Could you check a few things on this model? Use its own coordinates, in mm. A direction names the side the tool comes from. Round coordinates to 2 decimals unless told otherwise and drop trailing zeros. Loops run counter-clockwise (first coordinate to the right, second up) from the corner with the lowest first, then second, coordinate; pieces in that order, holes last. Notation, with made-up numbers: (44.5, -33.5) -> (70.5, -33.5) arc R14 cw to (70.5, -25.5) -> close; hole circle Ø10 at (-29, 57.25). An arc over 180 degrees is marked (long way). Put each result on its own line as item: value. Start each with the question number.
1. Imagine slicing it at B-B, the plane y = 20. Please give me the cut outline in (x, z), and give its area (3 significant figures).
2. I need wall thicknesses on line 1 (Y direction, x = 0, z = 0.5); line 2 (X direction, y = -3.5, z = 0.9); line 3 (X direction, y = 13.5, z = 0.7). Which ranges of each line are inside material? Lowest first, please. Write a range as [from, to].
3. I'm going to push a flat-ended pin straight in: P1, Ø4, axis at x = -11.76, y = -16.18, coming from the -Z side. Where does the tip first touch, or does it pass through?
4. Imagine slicing it at D-D, the plane z = 0.6. Count the separate pieces of the cut face and the enclosed holes in it, and give its area (3 significant figures).
5. If we mould it in two halves opening along X, with no side actions, what happens to faces 5 (the cylindrical face through (-17.156, -12.788, 0.493)), 6 (the cylindrical face through (17.369, 12.376, 0.493)), 7 (the cylindrical face through (6.363, 20.43, 0.493))? For each: pulls with the +X half, pulls with the -X half, needs draft (parallel to the pull), parting line crosses it, or undercut.
6. Which directions (+Z, -Z, +X, -X, +Y, -Y) give clear straight access to the entire face, cutting with the end or side of a thin tool? Please do faces 1 (the cylindrical face through (-17.464, 12.365, 0.493)), 2 (the flat face through (-6.925, 27.045, 0.493)), 3 (the flat face through (10.33, -26.04, 0.49)), 4 (the flat face through (6.95, 27.14, 0.49)).
7. Imagine slicing it at A-A, the plane x = 0. Please give me the cut outline in (y, z), and give its area (3 significant figures).
8. Imagine slicing it at C-C, the plane x = 22.5. Please give me the cut outline in (y, z), and give its area (3 significant figures).
```python
from build123d import *

# Parameters (mm, degrees)
SKETCH_1_R      = 12.9
SKETCH_1_R_2    = 1.5
EXTRUDE_1_DEPTH = 1


with BuildPart() as part:
    # 草图1 → 凸台-拉伸1 (new body)
    with BuildSketch(Plane.XY):
        with BuildLine():
            Line((-24.208730048, -20.05461018), (-18.863150132, -15.626310092))
            ThreePointArc((-18.863150132, -15.626310092), (-17.146898547, -12.74106365), (-17.642285858, -9.420708556))
            ThreePointArc((-17.642285858, -9.420708556), (-19.021130326, -6.180339887), (-19.810262634, -2.748362124))
            ThreePointArc((-19.810262634, -2.748362124), (-21.361141637, 0.229042931), (-24.445523644, 1.554468964))
            Line((-24.445523644, 1.554468964), (-31.373078125, 1.994985952))
            ThreePointArc((-31.373078125, 1.994985952), (-32.788486399, 2.717684101), (-33.230039203, 4.244348542))
            ThreePointArc((-33.230039203, 4.244348542), (-31.860393296, 10.352069312), (-29.378431918, 16.098376876))
            ThreePointArc((-29.378431918, 16.098376876), (-28.123857351, 17.073936127), (-26.55397669, 16.826655102))
            Line((-26.55397669, 16.826655102), (-20.690537997, 13.111126473))
            ThreePointArc((-20.690537997, 13.111126473), (-17.41615466, 12.370464403), (-14.41139241, 13.867651885))
            ThreePointArc((-14.41139241, 13.867651885), (-11.755705046, 16.180339888), (-8.735555524, 17.991388765))
            ThreePointArc((-8.735555524, 17.991388765), (-6.383123013, 20.386431107), (-6.075694405, 23.729431883))
            Line((-6.075694405, 23.729431883), (-7.797469917, 30.45405495))
            ThreePointArc((-7.797469917, 30.45405495), (-7.547528343, 32.023514221), (-6.232031499, 32.915221151))
            ThreePointArc((-6.232031499, 32.915221151), (0, 33.5), (6.232031499, 32.915221151))
            ThreePointArc((6.232031499, 32.915221151), (7.547528343, 32.023514221), (7.797469917, 30.45405495))
            Line((7.797469917, 30.45405495), (6.075694405, 23.729431883))
            ThreePointArc((6.075694405, 23.729431883), (6.383123013, 20.386431107), (8.735555524, 17.991388765))
            ThreePointArc((8.735555524, 17.991388765), (11.755705046, 16.180339887), (14.41139241, 13.867651885))
            ThreePointArc((14.41139241, 13.867651885), (17.41615466, 12.370464403), (20.690537997, 13.111126473))
            Line((20.690537997, 13.111126473), (26.55397669, 16.826655102))
            ThreePointArc((26.55397669, 16.826655102), (28.123857351, 17.073936127), (29.378431918, 16.098376876))
            ThreePointArc((29.378431918, 16.098376876), (31.860393296, 10.352069312), (33.230039203, 4.244348542))
            ThreePointArc((33.230039203, 4.244348542), (32.788486399, 2.717684101), (31.373078125, 1.994985952))
            Line((31.373078125, 1.994985952), (24.445523644, 1.554468964))
            ThreePointArc((24.445523644, 1.554468964), (21.361141637, 0.229042931), (19.810262634, -2.748362124))
            ThreePointArc((19.810262634, -2.748362124), (19.021130326, -6.180339888), (17.642285858, -9.420708556))
            ThreePointArc((17.642285858, -9.420708556), (17.146898547, -12.74106365), (18.863150132, -15.626310092))
            Line((18.863150132, -15.626310092), (24.208730048, -20.05461018))
            ThreePointArc((24.208730048, -20.05461018), (24.929028081, -21.471241373), (24.388900961, -22.965877077))
            ThreePointArc((24.388900961, -22.965877077), (19.690805952, -27.102069312), (14.305262176, -30.292069492))
            ThreePointArc((14.305262176, -30.292069492), (12.71687069, -30.343893076), (11.592158696, -29.221085825))
            Line((11.592158696, -29.221085825), (9.03247008, -22.768717229))
            ThreePointArc((9.03247008, -22.768717229), (6.818788557, -20.244874791), (3.50786011, -19.689969971))
            ThreePointArc((3.50786011, -19.689969971), (0, -20), (-3.50786011, -19.689969971))
            ThreePointArc((-3.50786011, -19.689969971), (-6.818788557, -20.244874791), (-9.03247008, -22.768717229))
            Line((-9.03247008, -22.768717229), (-11.592158696, -29.221085825))
            ThreePointArc((-11.592158696, -29.221085825), (-12.71687069, -30.343893076), (-14.305262176, -30.292069492))
            ThreePointArc((-14.305262176, -30.292069492), (-19.690805952, -27.102069312), (-24.388900961, -22.965877077))
            ThreePointArc((-24.388900961, -22.965877077), (-24.929028081, -21.471241373), (-24.208730048, -20.05461018))
        make_face()
        Circle(SKETCH_1_R, mode=Mode.SUBTRACT)
        with Locations((-11.755705046, -16.180339887)):
            Circle(SKETCH_1_R_2, mode=Mode.SUBTRACT)
        with Locations((-19.021130326, 6.180339888)):
            Circle(SKETCH_1_R_2, mode=Mode.SUBTRACT)
        with Locations((0, 20)):
            Circle(SKETCH_1_R_2, mode=Mode.SUBTRACT)
        with Locations((19.021130326, 6.180339887)):
            Circle(SKETCH_1_R_2, mode=Mode.SUBTRACT)
        with Locations((11.755705046, -16.180339888)):
            Circle(SKETCH_1_R_2, mode=Mode.SUBTRACT)
    extrude(amount=EXTRUDE_1_DEPTH)


solid = part.part
```
Entries:
1. outline: (-6.58, 0) -> (-1.5, 0) -> (-1.5, 1) -> (-6.58, 1) -> close; (1.5, 0) -> (6.58, 0) -> (6.58, 1) -> (1.5, 1) -> close
1. area: 10.2 mm^2
2. line 1: [-20, -12.9], [12.9, 18.5], [21.5, 33.5]
2. line 2: [-19.69, -12.42], [12.42, 19.69]
2. line 3: [-30.66, -21.3], [-14.81, 14.81], [21.3, 30.66]
3. P1: z = 0
4. separate pieces: 1
4. enclosed holes: 6
4. area: 1,630 mm^2
5. face 5: pulls with the -X half
5. face 6: undercut
5. face 7: pulls with the +X half
6. face 1: +Z, -Z, +Y
6. face 2: +Z, -Z, -X
6. face 3: +Z, -Z, -Y
6. face 4: +Z, -Z, +X
7. outline: (-20, 0) -> (-12.9, 0) -> (-12.9, 1) -> (-20, 1) -> close; (12.9, 0) -> (18.5, 0) -> (18.5, 1) -> (12.9, 1) -> close; (21.5, 0) -> (33.5, 0) -> (33.5, 1) -> (21.5, 1) -> close
7. area: 24.7 mm^2
8. outline: (-24.82, 0) -> (-18.64, 0) -> (-18.64, 1) -> (-24.82, 1) -> close; (1.02, 0) -> (14.26, 0) -> (14.26, 1) -> (1.02, 1) -> close
8. area: 19.4 mm^2
